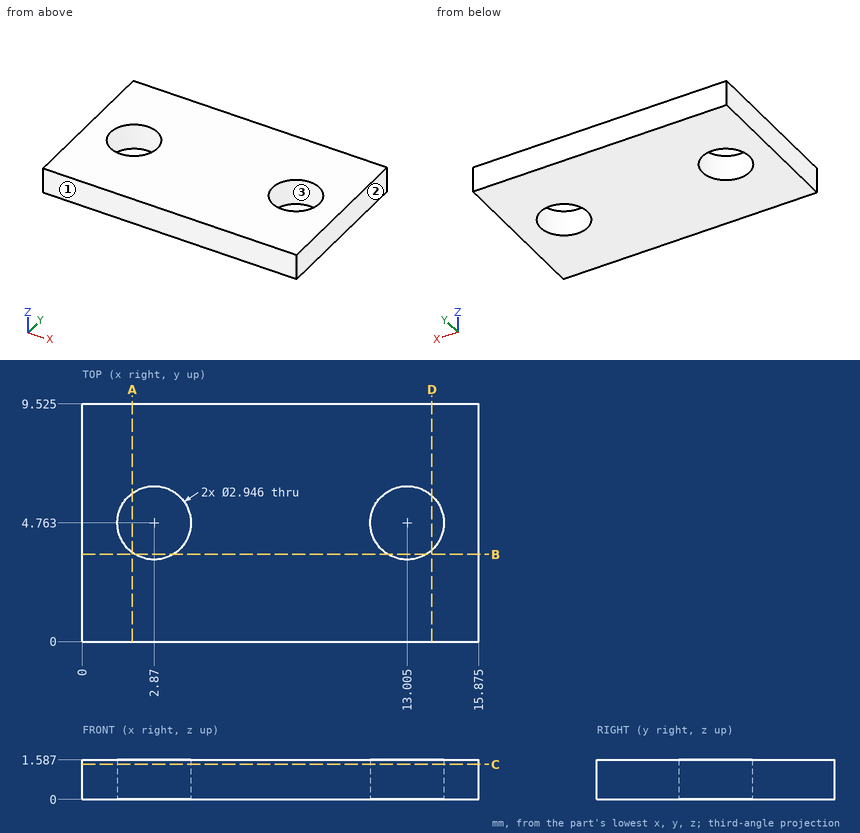
Geometry check sheet. Reference: drawing and pictorial views, mm from the part's lowest x, y, z. Coordinates: 2 decimals unless noted, no trailing zeros. Order: outer loops, then holes, each group sorted by start corner. A loop starts at its lowest first (then second) coordinate and runs counter-clockwise, first axis right, second up. Notation, with made-up numbers: (-19.75, 61.5) - (13.25, 61.5) arc R18 ccw to (13.25, 88.5) - close; hole circle Ø7 at (41, -3). An arc over 180 degrees is marked (long way). Answer in a Markdown table with one row per item. Add a question column.
1) Cross-section at A-A, the plane x = 2. Record the cut outline in (y, z) (1 decimal).
2) Cross-section at D-D, the plane x = 14. Record the cut outline in (y, z) (1 decimal).
3) Cross-section at B-B, the plane y = 3.5. Record the cut outline in (x, z) (1 decimal).
4) Cross-section at C-C, the plane z = 1.4. Record the cut outline in (x, y) (1 decimal).
5) Material ranges on line 1 along X through (y, z) = (4.5, 0.75) (1 decimal); line 2 along X through (y, z) = (4, 1.1) (1 decimal); line 3 along Y through (x, z) = (3.5, 0.25) (1 decimal), recorded low to high. Write a range as [from, to].
6) Release check for a two-part mould opening along X. For the marked faces 1, 2 and 3 record: +X half, -X half, draft (parallel to the pull), parting line (faces both ways), or undercut.
Check result:
| question | item | result |
|---|---|---|
| 1 | outline | (0, 0) - (3.6, 0) - (3.6, 1.6) - (0, 1.6) - close; (6, 0) - (9.5, 0) - (9.5, 1.6) - (6, 1.6) - close |
| 2 | outline | (0, 0) - (3.7, 0) - (3.7, 1.6) - (0, 1.6) - close; (5.8, 0) - (9.5, 0) - (9.5, 1.6) - (5.8, 1.6) - close |
| 3 | outline | (0, 0) - (2.1, 0) - (2.1, 1.6) - (0, 1.6) - close; (3.6, 0) - (12.2, 0) - (12.2, 1.6) - (3.6, 1.6) - close; (13.8, 0) - (15.9, 0) - (15.9, 1.6) - (13.8, 1.6) - close |
| 4 | outline | (0, 0) - (15.9, 0) - (15.9, 9.5) - (0, 9.5) - close; hole circle Ø2.9 at (2.9, 4.8); hole circle Ø2.9 at (13, 4.8) |
| 5 | line 1 | x = [0, 1.4], [4.3, 11.6], [14.5, 15.9] |
| 5 | line 2 | x = [0, 1.6], [4.1, 11.7], [14.3, 15.9] |
| 5 | line 3 | y = [0, 3.4], [6.1, 9.5] |
| 6 | face 1 | draft |
| 6 | face 2 | +X half |
| 6 | face 3 | undercut |
